```python
from build123d import *

# Parameters (mm, degrees)
EXTRUDE_1_DEPTH     = 2
SKETCH_2_R          = 6
EXTRUDE_2_DEPTH     = 1.5
SKETCH_3_R          = 5
EXTRUDE_3_DEPTH     = 4
SKETCH_4_R          = 5
EXTRUDE_4_DEPTH     = 1
SKETCH_5_R          = 4
EXTRUDE_5_DEPTH     = 3.5
CUT_EXTRUDE_1_DEPTH = 27.58006772
EXTRUDE_START       = -3.5
SKETCH_9_R          = 6
EXTRUDE_6_DEPTH     = 3.5
SKETCH_10_R         = 1.5
CUT_EXTRUDE_2_DEPTH = 26.029982022
CHAMFER_1_SIZE      = 1.7
CHAMFER_2_SIZE      = 0.5
CHAMFER_3_SIZE      = 0.5


with BuildPart() as part:
    # ｽｹｯﾁ1 → ﾎﾞｽ - 押し出し1 (new body)
    with BuildSketch(Plane.XY):
        with BuildLine():
            ThreePointArc((-6, 4.5), (0, -7.5), (6, 4.5))
            ThreePointArc((6, 4.5), (5, 7.5), (6, 10.5))
            ThreePointArc((6, 10.5), (0, 22.5), (-6, 10.5))
            ThreePointArc((-6, 10.5), (-5, 7.5), (-6, 4.5))
        make_face()
    extrude(amount=EXTRUDE_1_DEPTH)

    # ｽｹｯﾁ2 → ﾎﾞｽ - 押し出し2 (add)
    with BuildSketch(Plane.XY.offset(2)):
        with Locations(Location((0, 0, 0), (0, 0, 180))):
            Circle(SKETCH_2_R)
    extrude(amount=EXTRUDE_2_DEPTH)

    # ｽｹｯﾁ3 → ﾎﾞｽ - 押し出し3 (add)
    with BuildSketch(Plane.XY.offset(3.5)):
        Circle(SKETCH_3_R)
    extrude(amount=EXTRUDE_3_DEPTH)

    # ｽｹｯﾁ4 → ﾎﾞｽ - 押し出し4 (add)
    with BuildSketch(Plane(origin=(0, 0, 0), x_dir=(-1, 0, 0), z_dir=(0, 0, -1))):
        with Locations((0, 15)):
            Circle(SKETCH_4_R)
    extrude(amount=EXTRUDE_4_DEPTH)

    # ｽｹｯﾁ5 → ﾎﾞｽ - 押し出し5 (add)
    with BuildSketch(Plane(origin=(0, 0, -1), x_dir=(-1, 0, 0), z_dir=(0, 0, -1))):
        with Locations((0, 15)):
            Circle(SKETCH_5_R)
    extrude(amount=EXTRUDE_5_DEPTH)

    # ｽｹｯﾁ8 → ｶｯﾄ - 押し出し1 (cut, through all)
    with BuildSketch(Plane.XY.offset(7.5)):
        with BuildLine():
            ThreePointArc((-1.437472271, 3.928571429), (0, 2), (1.437472271, 3.928571429))
            ThreePointArc((1.437472271, 3.928571429), (1.590604363, 4.45051627), (2.12958855, 4.523809524))
            ThreePointArc((2.12958855, 4.523809524), (0, 5), (-2.12958855, 4.523809524))
            ThreePointArc((-2.12958855, 4.523809524), (-1.590604363, 4.45051627), (-1.437472271, 3.928571429))
        make_face()
        with BuildLine():
            ThreePointArc((4.120978793, -0.71939821), (1.732050808, -1), (2.683506522, -3.209173218))
            ThreePointArc((2.683506522, -3.209173218), (3.058957968, -3.602761921), (2.852939695, -4.106182546))
            ThreePointArc((2.852939695, -4.106182546), (4.330127019, -2.5), (4.982528245, -0.417626978))
            ThreePointArc((4.982528245, -0.417626978), (4.649562331, -0.847754349), (4.120978793, -0.71939821))
        make_face()
        with BuildLine():
            ThreePointArc((-2.683506522, -3.209173218), (-1.732050808, -1), (-4.120978793, -0.71939821))
            ThreePointArc((-4.120978793, -0.71939821), (-4.649562331, -0.847754349), (-4.982528245, -0.417626978))
            ThreePointArc((-4.982528245, -0.417626978), (-4.330127019, -2.5), (-2.852939695, -4.106182546))
            ThreePointArc((-2.852939695, -4.106182546), (-3.058957968, -3.602761921), (-2.683506522, -3.209173218))
        make_face()
    extrude(amount=-CUT_EXTRUDE_1_DEPTH, mode=Mode.SUBTRACT)

    # ｽｹｯﾁ9 → ﾎﾞｽ - 押し出し6 (add)
    with BuildSketch(Plane.XY.offset(3.5).offset(EXTRUDE_START)):
        with Locations(Location((0, 0, 0), (0, 0, 180))):
            Circle(SKETCH_9_R)
    extrude(amount=EXTRUDE_6_DEPTH)

    # ｽｹｯﾁ10 → ｶｯﾄ - 押し出し2 (cut, through all)
    with BuildSketch(Plane.XY.offset(3.5)):
        with Locations(Location((0, 3.5, 0), (0, 0, 16.601549599))):
            Circle(SKETCH_10_R)
        with Locations(Location((-3.031088913, -1.75, 0), (0, 0, 283.398450401))):
            Circle(SKETCH_10_R)
        with Locations(Location((3.031088913, -1.75, 0), (0, 0, 43.398450401))):
            Circle(SKETCH_10_R)
    extrude(amount=-CUT_EXTRUDE_2_DEPTH, mode=Mode.SUBTRACT)

    # 面取り1
    # the kernel refuses this chamfer: 1.7 mm, written as the material it takes off along each edge
    with BuildSketch(Plane(origin=(0, 3.5, 0), x_dir=(0.9583148475000108, 0.28571428571394725, 0), z_dir=(0.28571428571394725, -0.9583148475000108, 0))) as chamfer_1_piece_1:
        Polygon((1.5 + CHAMFER_1_SIZE, 0), (1.5, CHAMFER_1_SIZE), (1.5, 0), align=None)
    revolve(axis=Axis((0, 3.5, 0), (0, 0, 1)), mode=Mode.SUBTRACT)
    with BuildSketch(Plane(origin=(-3.031088913, -1.75, 0), x_dir=(0.2317215940976018, -0.9727821456157932, 0), z_dir=(-0.9727821456157932, -0.2317215940976018, 0))) as chamfer_1_piece_2:
        Polygon((1.5 + CHAMFER_1_SIZE, 0), (1.5, CHAMFER_1_SIZE), (1.5, 0), align=None)
    revolve(axis=Axis((-3.031088913, -1.75, 0), (0, 0, 1)), mode=Mode.SUBTRACT)
    with BuildSketch(Plane(origin=(3.031088913, -1.75, 0), x_dir=(0.7265932534024093, 0.6870678599018457, 0), z_dir=(0.6870678599018457, -0.7265932534024093, 0))) as chamfer_1_piece_3:
        Polygon((1.5 + CHAMFER_1_SIZE, 0), (1.5, CHAMFER_1_SIZE), (1.5, 0), align=None)
    revolve(axis=Axis((3.031088913, -1.75, 0), (0, 0, 1)), mode=Mode.SUBTRACT)

    # 面取り2
    chamfer_2_edges = [part.edges().sort_by_distance(p)[0] for p in [
        (4, 15, -4.5),
        (0, 22.5, 0),
        (5, 7.5, 0),
        (0, -7.5, 0),
        (-5, 7.5, 0),
    ]]
    chamfer(chamfer_2_edges, length=CHAMFER_2_SIZE)

    # 面取り3
    # the kernel refuses this chamfer: 0.5 mm, written as the material it takes off along each edge
    with BuildSketch(Plane(origin=(10, 7.5, 2), x_dir=(-0.7999999999999996, -0.6000000000000005, 0), z_dir=(0.6000000000000005, -0.7999999999999996, 0))) as chamfer_3_piece_1:
        Polygon((5, CHAMFER_3_SIZE), (5 + CHAMFER_3_SIZE, 0), (5, 0), align=None)
    revolve(axis=Axis((10, 7.5, 2), (0, 0, -1)), revolution_arc=73.739795292, mode=Mode.SUBTRACT)
    with BuildSketch(Plane(origin=(0, 15, 2), x_dir=(0.7999999999999998, -0.6000000000000002, 0), z_dir=(-0.6000000000000002, -0.7999999999999998, 0))) as chamfer_3_piece_2:
        Polygon((7.5 - CHAMFER_3_SIZE, 0), (7.5, -CHAMFER_3_SIZE), (7.5, 0), align=None)
    revolve(axis=Axis((0, 15, 2), (0, 0, 1)), revolution_arc=253.739795292, mode=Mode.SUBTRACT)
    with BuildSketch(Plane(origin=(0, 0, 7.5), x_dir=(-0.18173044344345904, 0.9833483848188515, 0), z_dir=(0.9833483848188515, 0.18173044344345904, 0))) as chamfer_3_piece_3:
        Polygon((5, -CHAMFER_3_SIZE), (5 - CHAMFER_3_SIZE, 0), (5, 0), align=None)
    revolve(axis=Axis((0, 0, 7.5), (0, 0, 1)), revolution_arc=99.05886102, mode=Mode.SUBTRACT)
    with BuildSketch(Plane(origin=(-10, 7.5, 2), x_dir=(0.8, 0.6, 0), z_dir=(-0.6, 0.8, 0))) as chamfer_3_piece_4:
        Polygon((5 + CHAMFER_3_SIZE, 0), (5, CHAMFER_3_SIZE), (5, 0), align=None)
    revolve(axis=Axis((-10, 7.5, 2), (0, 0, -1)), revolution_arc=73.739795292, mode=Mode.SUBTRACT)
    with BuildSketch(Plane(origin=(0, 0, 7.5), x_dir=(0.9424699037452493, -0.3342910117463833, 0), z_dir=(-0.3342910117463833, -0.9424699037452493, 0))) as chamfer_3_piece_5:
        Polygon((5, -CHAMFER_3_SIZE), (5 - CHAMFER_3_SIZE, 0), (5, 0), align=None)
    revolve(axis=Axis((0, 0, 7.5), (0, 0, 1)), revolution_arc=99.05886102, mode=Mode.SUBTRACT)
    with BuildSketch(Plane(origin=(0, 0, 7.5), x_dir=(-0.7607394603017978, -0.6490573730724652, 0), z_dir=(-0.6490573730724652, 0.7607394603017978, 0))) as chamfer_3_piece_6:
        Polygon((5, -CHAMFER_3_SIZE), (5 - CHAMFER_3_SIZE, 0), (5, 0), align=None)
    revolve(axis=Axis((0, 0, 7.5), (0, 0, 1)), revolution_arc=99.05886102, mode=Mode.SUBTRACT)
    with BuildSketch(Plane(origin=(0, 0, 2), x_dir=(-0.7999999999999997, 0.6000000000000003, 0), z_dir=(0.6000000000000003, 0.7999999999999997, 0))) as chamfer_3_piece_7:
        Polygon((7.5, -CHAMFER_3_SIZE), (7.5 - CHAMFER_3_SIZE, 0), (7.5, 0), align=None)
    revolve(axis=Axis((0, 0, 2), (0, 0, 1)), revolution_arc=253.739795292, mode=Mode.SUBTRACT)


solid = part.part
```
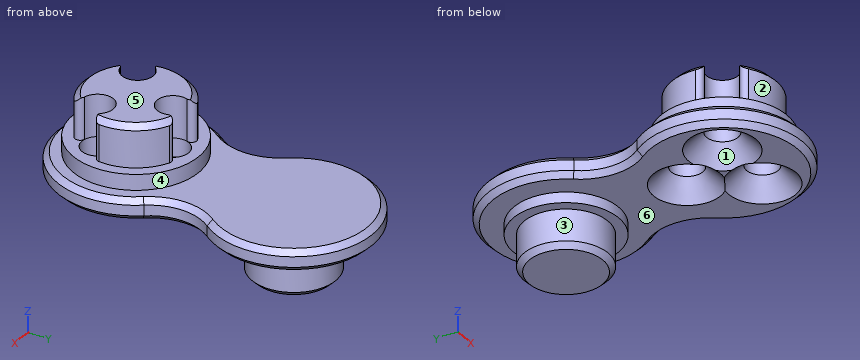
Part model, mm, in its own coordinate system. Face numbers are marked on the shaded views. A direction names the side the tool comes from. Round coordinates to 2 decimals unless told otherwise and drop trailing zeros. Order: outer loops, then holes, each group sorted by start corner. A loop starts at its lowest first (then second) coordinate and runs counter-clockwise, first axis right, second up. Notation, with made-up numbers: M 47,-16 L 52,-16 A13 ccw 52,4 Z; hole C 26,56 d5. An arc over 180 degrees is marked long. Put each result on its own line as item: value. Start each with the question number.
1. Slice it at B-B on y = -1.75. State how many separate pieces and enclosed holes the cut face has, then the cut area to 3 significant figures.
2. Slice it at A-A on z = -2.25. List the corners of the cut face in (x, y).
3. Drill centre lines: probe 1 along Y at (x, z) = (0, 2.45); probe 2 along X at (y, z) = (-1.75, 2.1); probe 3 along Z at (x, y) = (-5.75, 16.5). Where is each one in solid material? Low to high. Write a range as [from, to].
4. Two-plate mould, pull along Y, no slides. Class the marked faces 1, 2 and 3: +Y half, -Y half, draft (parallel to the pull), parting line (faces both ways), or undercut.
5. Drop flat-ended pins along their axis: pin 1 (3 mm diameter, centred on y = 12, z = 2, fed in from +X); pin 2 (1.8 mm diameter, centred on x = 0, y = 3.5, fed in from -Z); pin 3 (1 mm diameter, centred on x = -3, z = 2, fed in from -Y); pin 4 (0.9 mm diameter, centred on x = 0, y = 0, fed in from -Z). Give the stop position or say it passes through.
6. Tool access for the marked faces 4, 5 and 6: list every direction of +Z, -Z, +X, -X, +Y, -Y with a clear straight run to the whole face (end or side of a thin tool).
Findings:
1. separate pieces: 3
1. enclosed holes: 0
1. area: 31.4 mm2
2. outline: C 0,15 d8
3. probe 1: [-6, 2], [5, 6]
3. probe 2: [-5.74, -4.53], [-1.53, 1.53], [4.53, 5.74]
3. probe 3: [0, 2]
4. face 1: undercut
4. face 2: -Y half
4. face 3: parting line
5. pin 1: x = 7.33
5. pin 2: through
5. pin 3: y = -6.91
5. pin 4: z = 0
6. face 4: +Z
6. face 5: +Z, +X, -X, +Y, -Y
6. face 6: -Z
